The model under review builds one solid part; all positions refer to its coordinate system, in mm. A direction names the side the tool comes from. Round coordinates to 2 decimals unless told otherwise and drop trailing zeros. Order: outer loops, then holes, each group sorted by start corner. A loop starts at its lowest first (then second) coordinate and runs counter-clockwise, first axis right, second up.
```python
from build123d import *

# Parameters (mm, degrees)
EXTRUDE_1_DEPTH     = 61.6
SHELL_1_T           = -2
FILLET_2_R          = 3
CUT_EXTRUDE_1_REACH = 36
SKETCH_3_W          = 4.6
SKETCH_3_H          = 7.4
SKETCH_4_W          = 4.6
SKETCH_4_H          = 7.4
EXTRUDE_2_DEPTH     = 3.7
SKETCH_5_W          = 2.95
SKETCH_5_H          = 7.9
SKETCH_5_W_2        = 25.755
SKETCH_5_H_2        = 2
EXTRUDE_3_DEPTH     = 1
EXTRUDE_4_DEPTH     = 7.897587
CUT_EXTRUDE_START   = -61.6
CUT_EXTRUDE_3_DEPTH = 61.6
CUT_EXTRUDE_START_2 = -54.8
CUT_EXTRUDE_4_DEPTH = 54.8
CUT_EXTRUDE_5_DEPTH = 3.5
CUT_EXTRUDE_6_DEPTH = 3.5
CUT_EXTRUDE_START_3 = -2
CUT_EXTRUDE_7_DEPTH = 2
EXTRUDE_5_DEPTH     = 24.01


with BuildPart() as part:
    # ｽｹｯﾁ2 → ﾎﾞｽ - 押し出し1 (new body)
    with BuildSketch(Plane(origin=(0, 0, 0), x_dir=(0, 0, -1), z_dir=(1, 0, 0))):
        with BuildLine():
            Line((0, 0), (24, 0))
            ThreePointArc((24, 0), (31.071067812, 2.928932188), (34, 10))
            Line((34, 10), (34, 44.8))
            ThreePointArc((34, 44.8), (31.071067812, 51.871067812), (24, 54.8))
            Line((24, 54.8), (0, 54.8))
            Line((0, 54.8), (0, 0))
        make_face()
    extrude(amount=EXTRUDE_1_DEPTH)

    # ｼｪﾙ1
    shell_1_openings = [part.faces().sort_by_distance(p)[0] for p in [
        (30.8, 27.4, 0),
    ]]
    offset(amount=SHELL_1_T, openings=shell_1_openings, kind=Kind.INTERSECTION)

    # ﾌｨﾚｯﾄ2
    fillet_2_edges = [part.edges().sort_by_distance(p)[0] for p in [
        (61.6, 2.928932188, -31.071067812),
        (61.6, 27.4, -34),
        (61.6, 51.871067812, -31.071067812),
        (61.6, 54.8, -12),
        (0, 54.8, -12),
        (0, 51.871067812, -31.071067812),
        (0, 27.4, -34),
        (61.6, 0, -12),
        (0, 2.928932188, -31.071067812),
        (0, 0, -12),
    ]]
    fillet(fillet_2_edges, radius=FILLET_2_R)

    # ｽｹｯﾁ3 → ｶｯﾄ - 押し出し1 (cut, up to next)
    with BuildSketch(Plane(origin=(0, 0, -34), x_dir=(-1, 0, 0), z_dir=(0, 0, -1)), mode=Mode.PRIVATE) as cut_extrude_1_sk1:
        with Locations((-37.2975, 27.4)):
            Rectangle(SKETCH_3_W, SKETCH_3_H)
    cut_extrude_1_tool1 = extrude(cut_extrude_1_sk1.sketch, amount=-CUT_EXTRUDE_1_REACH, mode=Mode.PRIVATE) & part.part
    add(cut_extrude_1_tool1.solids().sort_by_distance((37.2975, 27.4, -34))[0], mode=Mode.SUBTRACT)
    # ｽｹｯﾁ3 → ｶｯﾄ - 押し出し1 (cut, up to next)
    with BuildSketch(Plane(origin=(0, 0, -34), x_dir=(-1, 0, 0), z_dir=(0, 0, -1)), mode=Mode.PRIVATE) as cut_extrude_1_sk2:
        with Locations((-24.3025, 27.4)):
            Rectangle(SKETCH_3_W, SKETCH_3_H)
    cut_extrude_1_tool2 = extrude(cut_extrude_1_sk2.sketch, amount=-CUT_EXTRUDE_1_REACH, mode=Mode.PRIVATE) & part.part
    add(cut_extrude_1_tool2.solids().sort_by_distance((24.3025, 27.4, -34))[0], mode=Mode.SUBTRACT)

    # ｽｹｯﾁ4 → ﾎﾞｽ - 押し出し2 (add)
    with BuildSketch(Plane.XY.offset(-34)):
        Polygon((17.9225, 15.575), (30.6725, 15.575), (43.6775, 15.575), (43.6775, 39.225), (30.6725, 39.225), (17.9225, 39.225), align=None)
        with Locations((24.3025, 27.4)):
            Rectangle(SKETCH_4_W, SKETCH_4_H, mode=Mode.SUBTRACT)
        with Locations((37.2975, 27.4)):
            Rectangle(SKETCH_4_W, SKETCH_4_H, mode=Mode.SUBTRACT)
    extrude(amount=EXTRUDE_2_DEPTH)

    # ｽｹｯﾁ5 → ﾎﾞｽ - 押し出し3 (add)
    with BuildSketch(Plane.XY.offset(-30.3)):
        with Locations((19.3975, 27.4)):
            Rectangle(SKETCH_5_W, SKETCH_5_H)
        with Locations((42.2025, 27.4)):
            Rectangle(SKETCH_5_W, SKETCH_5_H)
        with Locations((30.8, 38.225)):
            Rectangle(SKETCH_5_W_2, SKETCH_5_H_2)
        with Locations((30.8, 16.575)):
            Rectangle(SKETCH_5_W_2, SKETCH_5_H_2)
    extrude(amount=EXTRUDE_3_DEPTH)

    # ｽｹｯﾁ6 → ﾎﾞｽ - 押し出し4 (add)
    with BuildSketch(Plane(origin=(-6.518280687, 23.45241299, -44.223812227), x_dir=(1, 0, 0), z_dir=(0, 1, 0))):
        Polygon((34.190780687, -13.923812227), (40.445780687, -13.923812227), (40.445780687, -21.323812227), (42.170780687, -21.323812227), (42.170780687, -24.323812227), (32.465780687, -24.323812227), (32.465780687, -21.323812227), (34.190780687, -21.323812227), align=None)
    extrude(amount=EXTRUDE_4_DEPTH)

    # ｽｹｯﾁ8 → ｶｯﾄ - 押し出し3 (cut)
    with BuildSketch(Plane.ZY.offset(CUT_EXTRUDE_START)):
        with BuildLine():
            Line((0, 51.399152482), (0, 39.600847518))
            ThreePointArc((0, 39.600847518), (-3, 45.5), (0, 51.399152482))
        make_face()
        with BuildLine():
            Line((0, 15.199152482), (0, 3.400847518))
            ThreePointArc((0, 3.400847518), (-3, 9.3), (0, 15.199152482))
        make_face()
    extrude(amount=CUT_EXTRUDE_3_DEPTH, mode=Mode.SUBTRACT)

    # ｽｹｯﾁ9 → ｶｯﾄ - 押し出し4 (cut)
    with BuildSketch(Plane.XZ.offset(CUT_EXTRUDE_START_2)):
        with BuildLine():
            Line((56.299152482, 0), (44.500847518, 0))
            ThreePointArc((44.500847518, 0), (50.4, -3), (56.299152482, 0))
        make_face()
        with BuildLine():
            Line((17.099152482, 0), (5.300847518, 0))
            ThreePointArc((5.300847518, 0), (11.2, -3), (17.099152482, 0))
        make_face()
    extrude(amount=CUT_EXTRUDE_4_DEPTH, mode=Mode.SUBTRACT)

    # ｽｹｯﾁ11 → ｶｯﾄ - 押し出し5 (cut, symmetric)
    with BuildSketch(Plane(origin=(0, 27.4, 0), x_dir=(-1, 0, 0), z_dir=(0, -1, 0))):
        Polygon((-59.6, 1.176601917), (-59.6, 2.476687437), (-60.288664164, 1.788023273), (-60.288664164, 1.176601917), align=None)
        Polygon((-1.311335836, 1.176601917), (-2, 1.176601917), (-2, 2.476687437), (-1.311335836, 1.788023273), align=None)
    extrude(amount=CUT_EXTRUDE_5_DEPTH, both=True, mode=Mode.SUBTRACT)

    # ｽｹｯﾁ12 → ｶｯﾄ - 押し出し6 (cut, symmetric)
    with BuildSketch(Plane(origin=(30.8, 0, 0), x_dir=(0, 0, -1), z_dir=(1, 0, 0))):
        Polygon((2.501421356, 2), (1.201335836, 2), (1.201335836, 1.311335836), (1.812757192, 1.311335836), align=None)
        Polygon((1.812757192, 53.488664164), (2.501421356, 52.8), (1.201335836, 52.8), (1.201335836, 53.488664164), align=None)
    extrude(amount=CUT_EXTRUDE_6_DEPTH, both=True, mode=Mode.SUBTRACT)

    # ｽｹｯﾁ13 → ｶｯﾄ - 押し出し7 (cut)
    with BuildSketch(Plane.XZ.offset(CUT_EXTRUDE_START_3)):
        with BuildLine():
            Line((15.396028325, 0), (15.396028325, -12.526786251))
            ThreePointArc((15.396028325, -12.526786251), (13.821186559, -17.758317958), (18.796028325, -15.5))
            Line((18.796028325, -15.5), (18.796028325, 0))
            Line((18.796028325, 0), (15.396028325, 0))
        make_face()
        with BuildLine():
            Line((46.203971675, 0), (42.803971675, 0))
            Line((42.803971675, 0), (42.803971675, -15.5))
            ThreePointArc((42.803971675, -15.5), (47.778813441, -17.758317958), (46.203971675, -12.526786251))
            Line((46.203971675, -12.526786251), (46.203971675, 0))
        make_face()
    extrude(amount=CUT_EXTRUDE_7_DEPTH, mode=Mode.SUBTRACT)

    # ｽｹｯﾁ14 → ﾎﾞｽ - 押し出し5 (add)
    with BuildSketch(Plane.ZY.offset(-18.796028325)):
        with BuildLine():
            Line((-12.5, 2), (-18.5, 2))
            ThreePointArc((-18.5, 2), (-15.5, 5), (-12.5, 2))
        make_face()
    extrude(amount=-EXTRUDE_5_DEPTH)


solid = part.part
```
(1) To check wall thickness, follow probe 1 along X at (y, z) = (3, -7); probe 2 along Y at (x, z) = (54, -9); probe 3 along X at (y, z) = (1.15, -15.5). State the ranges of each line that lie inside material, in increasing order.
Data:
probe 1: x = 0 to 2, 59.6 to 61.6
probe 2: y = 0 to 2, 52.8 to 54.8
probe 3: x = 0.64 to 12.8, 18.8 to 42.8, 48.8 to 60.96
(2) Consider section C-C (x = 52). Write out the cut boundary in (y, z).
Data:
outline: (0, -24) arc R10 ccw to (10, -34) - (44.8, -34) arc R10 ccw to (54.8, -24) - (54.8, -2.82) - (52.8, -2.82) - (52.8, -24) arc R8 cw to (44.8, -32) - (10, -32) arc R8 cw to (2, -24) - (2, -2.82) - (0, -2.82) - close
(3) For faces 4 (the cylindrical face through (1, 9.2, -3)), 5 (the flat face through (33.928, 27, -27)), 6 (the flat face through (31, 17, -29.3)), list the 3-axis set-ups (+Z, -Z, +X, -X, +Y, -Y) from which the entire face can be reached by the end or side of a thin tool; tool diameter is ignored.
Data:
face 4: +Z, +X, -X
face 5: none
face 6: +Z
(4) Insertion check: pin 1 (1.5 mm diameter, centred on x = 45.5, y = 11, fed in from +Z); pin 2 (2.5 mm diameter, centred on x = 41.5, y = 26, fed in from +Z); pin 3 (0.6 mm diameter, centred on x = 32, y = 53, fed in from -Z). Each pin has a flat end and moves straight along its axis. Give the tip position at first contact, or say it passes through.
Data:
pin 1: stops at z = -32
pin 2: stops at z = -29.3
pin 3: stops at z = -30.13
(5) Consider section A-A (z = -21). Write out the cut boundary in (x, y), and give its area (3 significant figures).
Data:
outline: (0, 3) arc R3 ccw to (3, 0) - (58.6, 0) arc R3 ccw to (61.6, 3) - (61.6, 51.8) arc R3 ccw to (58.6, 54.8) - (3, 54.8) arc R3 ccw to (0, 51.8) - close; (25.95, 23.45) - (35.65, 23.45) - (35.65, 31.35) - (25.95, 31.35) - close; hole (2, 2) - (59.6, 2) - (59.6, 52.8) - (2, 52.8) - close
area: 519 mm2
(6) Draft analysis for pull direction Z (two halves, no side actions). For faces 1 (the flat face through (31, 1, 0)), 2 (the flat face through (31, 23.452, -24)), 3 (the cylindrical face through (13.75, 1.014, -17.694)), state which applies: pulls with the +Z half, pulls with the -Z half, needs draft (parallel to the pull), parting line crosses it, or undercut.
Data:
face 1: pulls with the +Z half
face 2: needs draft
face 3: undercut
(7) Consider section B-B (x = 38). Write out the cut boundary in (y, z) (3 decimals).
Data:
outline: (0, -24) arc R10 ccw to (10, -34) - (23.7, -34) - (23.7, -30.3) - (17.575, -30.3) - (17.575, -29.3) - (15.575, -29.3) - (15.575, -32) - (10, -32) arc R8 cw to (2, -24) - (2, -18.5) arc R3 ccw to (2, -12.5) - (2, 0) - (0, 0) - close; (31.1, -34) - (44.8, -34) arc R10 ccw to (54.8, -24) - (54.8, 0) - (52.8, 0) - (52.8, -24) arc R8 cw to (44.8, -32) - (39.225, -32) - (39.225, -29.3) - (37.225, -29.3) - (37.225, -30.3) - (31.1, -30.3) - close
